Can you work these out from the model? Positions are in its coordinate system, mm. A direction names the side the tool comes from. Give positions to 0.01 mm unless a question says otherwise; leave off trailing zeros. Order: outer loops, then holes, each group sorted by start corner. A loop starts at its lowest first (then second) coordinate and runs counter-clockwise, first axis right, second up. Notation, with made-up numbers: M 40.25,68 L 62.25,68 A10 cw 62.25,76 Z; hole C 74,-4.5 d11. An arc over 180 degrees is marked long. Answer as a JSON object with one key per item and string values.
```python
from build123d import *

# Parameters (mm, degrees)
F0_W      = 76.2
F0_H      = 12.7
F1_DEPTH  = 38.1
F4_DEPTH  = 19.05
F5_DEPTH  = 19.05
F6_R      = 9.525
F7_DEPTH  = 127
F8_R      = 12.7
F9_DEPTH  = 12.7
F10_R     = 12.7
F10_R_2   = 9.525
F11_DEPTH = 6.35


with BuildPart() as f1:
    # F0 (on Front) → F1 (new body)
    with BuildSketch(Plane.XZ):
        with Locations((38.1, 6.35)):
            Rectangle(F0_W, F0_H)
    extrude(amount=-F1_DEPTH)

    # F2 (on face) → F4 (join)
    with BuildSketch(Plane.XY.offset(12.7)):
        with BuildLine():
            ThreePointArc((38.1, 0), (51.570384, 5.579616), (57.15, 19.05))
            ThreePointArc((57.15, 19.05), (51.570384, 32.520384), (38.1, 38.1))
            ThreePointArc((38.1, 38.1), (19.05, 19.05), (38.1, 0))
        make_face()
    extrude(amount=F4_DEPTH)

    # F3 (on face) → F5 (join)
    with BuildSketch(Plane(origin=(0, 0, 0), x_dir=(1, 0, 0), z_dir=(0, 0, -1))):
        with BuildLine():
            ThreePointArc((38.1, -38.1), (51.570384, -32.520384), (57.15, -19.05))
            ThreePointArc((57.15, -19.05), (51.570384, -5.579616), (38.1, 0))
            ThreePointArc((38.1, 0), (19.05, -19.05), (38.1, -38.1))
        make_face()
    extrude(amount=F5_DEPTH)

    # F6 (on face) → F7 (cut)
    with BuildSketch(Plane.XY.offset(31.75)):
        with Locations((38.1, 19.05)):
            Circle(F6_R)
    extrude(amount=-F7_DEPTH, mode=Mode.SUBTRACT)

    # F8 (on face) → F9 (cut)
    with BuildSketch(Plane.XY.offset(31.75)):
        with Locations((38.1, 19.05)):
            Circle(F8_R)
    extrude(amount=-F9_DEPTH, mode=Mode.SUBTRACT)

    # F10 (on face) → F11 (join)
    with BuildSketch(Plane.XY.offset(31.75)):
        with Locations((38.1, 19.05)):
            Circle(F10_R)
        with Locations((38.1, 19.05)):
            Circle(F10_R_2, mode=Mode.SUBTRACT)
    extrude(amount=-F11_DEPTH)


solid = f1.part
```
1) I need wall thicknesses on L1, parallel to Y at x = 38.1, z = 22.5; L2, parallel to X at y = 19, z = 21; L3, parallel to X at y = 19, z = -1. Which ranges of each line are inside material? Lowest first, please.
Results found:
{"L1": "y = 0 to 6.35, 31.75 to 38.1", "L2": "x = 19.05 to 25.4, 50.8 to 57.15", "L3": "x = 19.05 to 28.58, 47.62 to 57.15"}
2) I want a section at B-B on x = 35. Write out the boundary of the cut face in (y, z), and give its area (3 significant figures).
Results found:
{"outline": "M 0,0 L 0.25,0 L 0.25,-19.05 L 10.04,-19.05 L 10.04,19.05 L 6.73,19.05 L 6.73,25.4 L 10.04,25.4 L 10.04,31.75 L 0.25,31.75 L 0.25,12.7 L 0,12.7 Z; M 28.06,-19.05 L 37.85,-19.05 L 37.85,0 L 38.1,0 L 38.1,12.7 L 37.85,12.7 L 37.85,31.75 L 28.06,31.75 L 28.06,25.4 L 31.37,25.4 L 31.37,19.05 L 28.06,19.05 Z", "area": "959 mm²"}
3) I want a section at C-C on z = -13. Write out the boundary of the cut face in (x, y) (3 decimals), and give its area (3 significant figures).
Results found:
{"outline": "C 38.1,19.05 d38.1; hole C 38.1,19.05 d19.05", "area": "855 mm²"}
4) For faces 5 (the face through (65, 19, 0)), 6 (the face through (49.832, 14.186, 22.269)), 7 (the face through (65, 19, 12.7)), which set-ups out of +Z, -Z, +X, -X, +Y, -Y let a thin tool reach every point of the face, with its end or its side?
Results found:
{"face 5": "-Z, +X", "face 6": "none", "face 7": "+Z, +X"}
5) I want a section at A-A on y = 25. Write out the boundary of the cut face in (x, z).
Results found:
{"outline": "M 0,0 L 20,0 L 20,-19.05 L 30.66,-19.05 L 30.66,19.05 L 26.88,19.05 L 26.88,25.4 L 30.66,25.4 L 30.66,31.75 L 20,31.75 L 20,12.7 L 0,12.7 Z; M 45.54,-19.05 L 56.2,-19.05 L 56.2,0 L 76.2,0 L 76.2,12.7 L 56.2,12.7 L 56.2,31.75 L 45.54,31.75 L 45.54,25.4 L 49.32,25.4 L 49.32,19.05 L 45.54,19.05 Z"}
6) I'm going to push flat-ended pins straight in: pin 1 Ø10 at (x, y) = (18, 12) entering from +Z; pin 2 Ø8 at (y, z) = (25.5, 22.5) entering from -X; pin 3 Ø4 at (x, y) = (9.5, 13.5) entering from -Z; pin 4 Ø4 at (y, z) = (8.5, 19.5) entering from -X. Where does each tip first touch, or does it pass through?
Results found:
{"pin 1": "stops at z = 31.75", "pin 2": "stops at x = 19.21", "pin 3": "stops at z = 0", "pin 4": "stops at x = 21.08"}
7) Thinking about a two-plate mould opening in Y: for faces 1 (the face through (30.541, 13.254, 0.267)), 2 (the face through (40, 29, 25.4)), 3 (the face through (10, 19, 0)), 4 (the face through (38, 0, 6)), which applies, pulls with the +Y half, pulls with the -Y half, needs draft (parallel to the pull), parting line crosses it, or undercut?
Results found:
{"face 1": "undercut", "face 2": "undercut", "face 3": "needs draft", "face 4": "pulls with the -Y half"}
8) I want a section at D-D on x = 70. Write out the boundary of the cut face in (y, z), and give its area (3 significant figures).
Results found:
{"outline": "M 0,0 L 38.1,0 L 38.1,12.7 L 0,12.7 Z", "area": "484 mm²"}
